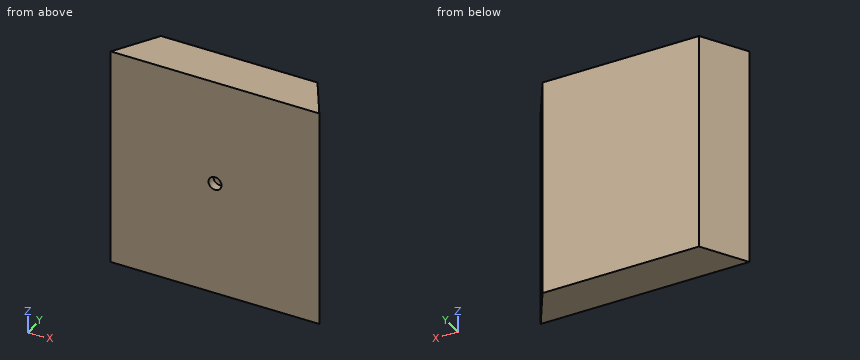
```python
from build123d import *

# Parameters (mm, degrees)
BOSS_EXTRUDE1_DEPTH = 250
SKETCH2_R           = 7.5
CUT_EXTRUDE1_DEPTH  = 10


with BuildPart() as part:
    # Sketch1 → Boss-Extrude1 (new body)
    with BuildSketch(Plane.XY):
        Polygon((-120, 0), (120, 0), (90, 50), (-90, 50), align=None)
    extrude(amount=-BOSS_EXTRUDE1_DEPTH)

    # Sketch2 → Cut-Extrude1 (cut)
    with BuildSketch(Plane.XZ):
        with Locations(Location((0, -120, 0), (0, 0, 270))):
            Circle(SKETCH2_R)
    extrude(amount=-CUT_EXTRUDE1_DEPTH, mode=Mode.SUBTRACT)


solid = part.part
```
Check sheet for the modelled part. Datum: model origin and axes. Units: mm. Coordinates: 2 decimals unless noted, no trailing zeros. Loops run counter-clockwise (first coordinate to the right, second up) from the corner with the lowest first, then second, coordinate; pieces in that order, holes last.
1) Sectioned sample at C-C (y = 23.5). Record the boundary of the cut face in (x, z).
2) Sectioned sample at B-B (z = -120). Record the boundary of the cut face in (x, y), and give its area (4 significant figures).
3) Sectioned sample at A-A (y = 5). Record the boundary of the cut face in (x, z).
4) Sectioned sample at D-D (x = -99.5). Record the boundary of the cut face in (y, z).
5) Gauge pin test, flat ends, axial feed: pin 1 (12 mm diameter, centred on y = 18, z = -220, fed in from -X); pin 2 (5 mm diameter, centred on y = 25.5, z = -146, fed in from +X). Record the tip position at first contact, or that the pin passes through.
6) Material ranges on probe 1 along X at (y, z) = (7.5, -120); probe 2 along X at (y, z) = (4, -120); probe 3 along X at (y, z) = (16, -160), recorded low to high.
Check sheet entries:
1. outline: (-105.9, -250) - (105.9, -250) - (105.9, 0) - (-105.9, 0) - close
2. outline: (-120, 0) - (-7.5, 0) - (-7.5, 10) - (7.5, 10) - (7.5, 0) - (120, 0) - (90, 50) - (-90, 50) - close
2. area: 10,350 mm2
3. outline: (-117, -250) - (117, -250) - (117, 0) - (-117, 0) - close; hole circle Ø15 at (0, -120)
4. outline: (0, -250) - (34.17, -250) - (34.17, 0) - (0, 0) - close
5. pin 1: stops at x = -112.8
5. pin 2: stops at x = 106.2
6. probe 1: x = -115.5 to -7.5, 7.5 to 115.5
6. probe 2: x = -117.6 to -7.5, 7.5 to 117.6
6. probe 3: x = -110.4 to 110.4
